For this review, take the finished solid that the model builds, in its own axes (mm). A direction names the side the tool comes from. Coordinates: 2 decimals unless noted, no trailing zeros. Write each loop counter-clockwise with the first axis right and the second up, starting at its lowest first coordinate (ties: lowest second). Pieces come first, ordered by that corner, then holes.
1) We need section B-B on y = -14. Write out the cut boundary in (x, z), then the cut area to 3 significant figures.
2) For faces 5 (the face through (-13, 14.5, -5)), 6 (the face through (13, -23, 0)), 7 (the face through (-8.5, 14.5, 0)), 8 (the face through (-2, 0, 0)), list the 3-axis set-ups (+Z, -Z, +X, -X, +Y, -Y) from which the entire face can be reached by the end or side of a thin tool; tool diameter is ignored.
3) We need section D-D on x = 16.5. Write out the cut boundary in (y, z), then the cut area to 3 significant figures.
4) To check wall thickness, follow line 1 along Y through (x, z) = (11, -5.25); line 2 along X through (y, z) = (-1, 3.5); line 3 along Y through (x, z) = (18.5, -0.5). State the ranges of each line that lie inside material, in increasing order.
5) Mouldability with a two-part tool opening along Y and no side actions: class faces 1 (the face through (0, -19, -7.5)), 2 (the face through (-13, 14.5, 5)), 3 (the face through (-13, 15, 0)), 4 (the face through (-10.81, -16.74, 0.11)) as pulls with the +Y half, pulls with the -Y half, needs draft (parallel to the pull), parting line crosses it, or undercut.
6) We need section A-A on z = -5.75. Write out the cut boundary in (x, y).
7) Insertion check: P1, Ø2, axis at x = -9.5, z = 5.5, coming from the +Y side; P2, Ø4, axis at y = 11.5, z = 1, coming from the +X side; P3, Ø0.6, axis at y = 14.5, z = -4.5, coming from the -X side; P4, Ø10, axis at x = 10.5, y = -9.5, coming from the -Z side. Each pin has a flat end and moves straight along its axis. Give the tip position at first contact, or say it passes through.
8) We need section C-C on z = -0.5. Write out the cut boundary in (x, y).
Autodesk Inventor part; units mm, degrees
ref_plane "YZ Plane" through (0, 0, 0) normal (1, 0, 0) x (0, 1, 0)
ref_plane "XZ Plane" through (0, 0, 0) normal (0, 1, 0) x (-1, 0, 0)
ref_plane "XY Plane" through (0, 0, 0) normal (0, 0, 1) x (1, 0, 0)
sketch "Sketch1" plane through (0, 0, 0) normal (0, 1, 0) x (-1, 0, 0)
  line L0 (-20, -7.5) -> (20, -7.5)
  line L1 (20, -7.5) -> (20, 7.5)
  line L2 (20, 7.5) -> (-20, 7.5)
  line L3 (-20, 7.5) -> (-20, -7.5)
  line L4 (-20, -7.5) -> (20, 7.5) construction
  line L5 (20, -7.5) -> (-20, 7.5) construction
  point P0 (0, 0)
  dimension "d0" = 15
  dimension "d1" = 40
extrude "Extrusion1" add sketch "Sketch1" along normal blind 5
sketch "Sketch2" plane through (20, 0, 7.5) normal (1, 0, 0) x (0, 0, -1)
  line L0 (15, 0) -> (0, 0)
  line L1 (0, -28) -> (0, 0)
  line L2 (15, 0) -> (15, -28)
  line L3 (15, -28) -> (0, -28)
  line L4 (0, 0) -> (15, 0)
  line L5 (15, 0) -> (0, 0)
  point P0 (7.5, 0)
  dimension "d13" = 28
extrude "Extrusion2" add sketch "Sketch2" against normal blind 5
sketch "Sketch3" plane through (-20, 5, 7.5) normal (0, 0, 1) x (1, 0, 0)
  line L0 (35, -5) -> (35, -33)
  line L1 (35, -33) -> (30, -33)
  line L2 (35, -28) -> (30, -28)
  line L3 (35, -25) -> (-4.3646, -25) construction
  line L4 (0, -5) -> (35, -5) construction
  line L5 (30, -33) -> (3.4423, -33)
  line L6 (35, -21) -> (-4.3646, -21) construction
  line L7 (3.4423, -33) -> (21.0714, -33)
  arc A0 (20.9558, -24.1562) -> (30, -28) centre (30.8945, -13.3333) ccw
  arc A1 (20.9558, -24.1562) -> (13.2077, -21) centre (12.838, -32.9961) ccw
  arc A2 (13.2077, -21) -> (5.7637, -24.1543) centre (12.91, -30.6583) ccw
  arc A3 (5.7637, -24.1543) -> (3.4423, -28) centre (11.7993, -30.4211) ccw
  line L8 (3.4423, -33) -> (3.4423, -28)
  point P0 (20, -5)
  point P1 (35, -5)
  dimension "d7" = 5
  dimension "d8" = 5
  dimension "d9" = 20
  dimension "d10" = 4
extrude "Extrusion3" add sketch "Sketch3" against normal up to surface (15 mm away)
sketch "Sketch4" plane through (0, 5, 0) normal (0, 1, 0) x (1, 0, 0)
  line L0 (-17.5, 4.25) -> (-9, 4.25)
  line L1 (-9, 4.25) -> (-9, -4.25)
  line L2 (-9, -4.25) -> (-17.5, -4.25)
  line L3 (-17.5, -4.25) -> (-17.5, 4.25)
  line L4 (-20, 7.5) -> (-20, -7.5)
  point P0 (0, 0)
  dimension "d14" = 8.5
  dimension "d15" = 2.5
  dimension "d16" = 4.25
  dimension "d17" = 4.25
extrude "Extrusion4" add sketch "Sketch4" along normal blind 10
sketch "Sketch5" plane through (0, 15, 0) normal (0, 1, 0) x (1, 0, 0)
  line L0 (-17.5, 4.25) -> (-9, 4.25)
  line L1 (-15.5, 4.25) -> (-11, 4.25)
  line L2 (-11, 4.25) -> (-11, 5.25)
  line L3 (-11, 5.25) -> (-15.5, 5.25)
  line L4 (-15.5, 5.25) -> (-15.5, 4.25)
  line L5 (-9, -4.25) -> (-9, 4.25)
  line L6 (-17.5, 4.25) -> (-17.5, -4.25)
  point P0 (0, 0)
  dimension "d20" = 2
  dimension "d21" = 2
  dimension "d22" = 1
extrude "Extrusion5" add sketch "Sketch5" against normal blind 0.5
sketch "Sketch6" plane through (0, 15, 0) normal (0, 1, 0) x (1, 0, 0)
  line L0 (-17.5, 4.25) -> (-9, 4.25) construction
  line L1 (-9, -4.25) -> (-9, 4.25) construction
  line L2 (-17.5, 4.25) -> (-9, -4.25) construction
  line L3 (-9, 4.25) -> (-17.5, -4.25) construction
  point P0 (0, 0)
  point P1 (-13.25, 0)
pattern_circular "Circular Pattern1" count 4 over 360 about axis through (-13.25, 15, 0) along (0, 1, 0) of "Extrusion5"
properties part number "GroundClipV1"
Result:
1. outline: (15, -7.5) - (20, -7.5) - (20, 7.5) - (15, 7.5) - close
1. area: 75.0 mm2
2. face 5: -Z, +X, -X
2. face 6: +Z, -Z
2. face 7: +Z, -Z, +X
2. face 8: +Z, -Z, -X
3. outline: (-28, -7.5) - (5, -7.5) - (5, 7.5) - (-28, 7.5) - close
3. area: 495 mm2
4. line 1: y = -28 to -23, 0 to 5
4. line 2: x = 15 to 20
4. line 3: y = -28 to 5
5. face 1: needs draft
5. face 2: undercut
5. face 3: pulls with the +Y half
5. face 4: undercut
6. outline: (-20, 0) - (15, 0) - (15, -23) - (10, -23) arc R14.69 cw to (0.96, -19.16) arc R12 ccw to (-6.79, -16) arc R9.66 ccw to (-14.24, -19.15) arc R8.7 ccw to (-16.56, -23) - (-16.56, -28) - (20, -28) - (20, 5) - (-20, 5) - close
7. P1: stops at y = 5
7. P2: stops at x = -9
7. P3: stops at x = -17.5
7. P4: stops at z = -7.5
8. outline: (-20, 0) - (15, 0) - (15, -23) - (10, -23) arc R14.69 cw to (0.96, -19.16) arc R12 ccw to (-6.79, -16) arc R9.66 ccw to (-14.24, -19.15) arc R8.7 ccw to (-16.56, -23) - (-16.56, -28) - (20, -28) - (20, 5) - (-9, 5) - (-9, 14.5) - (-8, 14.5) - (-8, 15) - (-18.5, 15) - (-18.5, 14.5) - (-17.5, 14.5) - (-17.5, 5) - (-20, 5) - close
